Geometry: final body of the model. Coordinates: model frame, mm. A direction names the side the tool comes from. Round coordinates to 2 decimals unless told otherwise and drop trailing zeros. Loops run counter-clockwise (first coordinate to the right, second up) from the corner with the lowest first, then second, coordinate; pieces in that order, holes last. Notation, with made-up numbers: M 76.25,67.25 L 87.25,67.25 A32 ccw 87.25,97.25 Z; hole C 70.25,-20 d6. An arc over 180 degrees is marked long. Write each question's results on one line, items separated by ' | '.
Autodesk Inventor part; units mm, degrees
ref_plane "YZ Plane" through (0, 0, 0) normal (1, 0, 0) x (0, 1, 0)
ref_plane "XZ Plane" through (0, 0, 0) normal (0, 1, 0) x (-1, 0, 0)
ref_plane "XY Plane" through (0, 0, 0) normal (0, 0, 1) x (1, 0, 0)
sketch "Эскиз1" plane through (0, 0, 0) normal (0, 0, 1) x (1, 0, 0)
  line L0 (32.4057, 38.6485) -> (-32.4072, 38.6485)
  arc A0 (-32.4072, 38.6485) -> (-37.4072, 33.6485) centre (-32.4072, 33.6485) ccw
  line L1 (-37.4072, 33.6485) -> (-37.4072, 5)
  arc A1 (-37.4072, 5) -> (-32.4072, 0) centre (-32.4072, 5) ccw
  line L2 (-30, 0) -> (-29.5804, 0)
  arc A2 (-24.6503, -4.1667) -> (-29.5804, 0) centre (-29.5804, -5) ccw
  arc A3 (-24.6503, -4.1667) -> (24.6503, -4.1667) centre (0, 0) ccw
  arc A4 (29.5804, 0) -> (24.6503, -4.1667) centre (29.5804, -5) ccw
  circle A5 centre (0, 0) radius 13.45
  line L3 (-0.0007, 35) -> (-0.0007, -40.0249) construction
  line L4 (-31.1692, 11.8598) -> (-24.8192, 11.8598)
  line L5 (-24.8192, 11.8598) -> (-24.8192, 31.7098)
  line L6 (-24.8192, 31.7098) -> (-31.1692, 31.7098)
  line L7 (-31.1692, 31.7098) -> (-31.1692, 11.8598)
  line L8 (24.8177, 11.8598) -> (31.1677, 11.8598)
  line L9 (31.1677, 11.8598) -> (31.1677, 31.7098)
  line L10 (31.1677, 31.7098) -> (24.8177, 31.7098)
  line L11 (24.8177, 31.7098) -> (24.8177, 11.8598)
  arc A6 (37.4057, 33.6485) -> (32.4057, 38.6485) centre (32.4057, 33.6485) ccw
  line L12 (37.4057, 33.6485) -> (37.4057, 5)
  arc A7 (32.4057, 0) -> (37.4057, 5) centre (32.4057, 5) ccw
  line L13 (32.4057, 0) -> (29.5804, 0)
  line L14 (-32.4072, 0) -> (-30, 0)
  point P0 (29.9986, 30)
  point P1 (-30, 30)
  point P2 (25.9869, 30)
extrude "Выдавливание1" add sketch "Эскиз1" along normal blind 5
properties part number "Гор. шарнир"
1. Section A-A (x = 0). Output: boundary loops of the cut face in (y, z), then the cut area to 3 significant figures.
Answer key:
outline: M -25,0 L -13.45,0 L -13.45,5 L -25,5 Z; M 13.45,0 L 38.65,0 L 38.65,5 L 13.45,5 Z | area: 184 mm²
2. Section D-D (y = -11.5). Output: boundary loops of the cut face in (x, z), then the cut area to 3 significant figures.
Answer key:
outline: M -22.2,0 L -6.98,0 L -6.98,5 L -22.2,5 Z; M 6.98,0 L 22.2,0 L 22.2,5 L 6.98,5 Z | area: 152 mm²
3. Section C-C (y = 22). Output: boundary loops of the cut face in (x, z), then the cut area to 3 significant figures.
Answer key:
outline: M -37.41,0 L -31.17,0 L -31.17,5 L -37.41,5 Z; M -24.82,0 L 24.82,0 L 24.82,5 L -24.82,5 Z; M 31.17,0 L 37.41,0 L 37.41,5 L 31.17,5 Z | area: 311 mm²
4. Ray query, probe 1 along X at (y, z) = (29, 3.5); probe 2 along Y at (x, z) = (0, 3.5); probe 3 along Y at (x, z) = (5.5, 4.05). Return the intervals inside material, ascending.
Answer key:
probe 1: x = -37.41 to -31.17, -24.82 to 24.82, 31.17 to 37.41 | probe 2: y = -25 to -13.45, 13.45 to 38.65 | probe 3: y = -24.39 to -12.27, 12.27 to 38.65
5. Draft query along Y for faces 1 (the face through (35.902, 37.223, 2.465)), 2 (the face through (35.98, 1.504, 2.465)), 3 (the face through (31.168, 22, 2)). Return one class per face: pulls with the +Y half, pulls with the -Y half, needs draft (parallel to the pull), parting line crosses it, or undercut.
Answer key:
face 1: pulls with the +Y half | face 2: pulls with the -Y half | face 3: undercut
6. Section B-B (z = 4.1). Output: boundary loops of the cut face in (x, y), then the cut area to 3 significant figures.
Answer key:
outline: M -37.41,5 A5 ccw -32.41,0 L -29.58,0 A5 cw -24.65,-4.17 A25 ccw 24.65,-4.17 A5 cw 29.58,0 L 32.41,0 A5 ccw 37.41,5 L 37.41,33.65 A5 ccw 32.41,38.65 L -32.41,38.65 A5 ccw -37.41,33.65 Z; hole M -31.17,11.86 L -24.82,11.86 L -24.82,31.71 L -31.17,31.71 Z; hole C 0,0 d26.9; hole M 24.82,11.86 L 31.17,11.86 L 31.17,31.71 L 24.82,31.71 Z | area: 3,040 mm²
7. Access query for faces 4 (the face through (28, 31.71, 2)), 5 (the face through (-31, 0, 2)), 6 (the face through (31, 0, 2)). Directions: +Z, -Z, +X, -X, +Y, -Y. A direction counts if a zero-diameter tool reaches every point of the face in a straight line with its end or side. Return the directions, or none.
Answer key:
face 4: +Z, -Z | face 5: +Z, -Z, -X, -Y | face 6: +Z, -Z, +X, -Y
8. Pin query (flat end, axial travel): P1, Ø1.5, axis at x = -29, z = 2, coming from the -Y side; P2, Ø1.5, axis at x = 28, z = 2.5, coming from the -Y side; P3, Ø1, axis at y = -13, z = 3, coming from the +X side; P4, Ø24, axis at x = 0, y = 0, coming from the +Z side. Return the tip coordinate at first contact, or that it passes through.
Answer key:
P1: stops at y = -0.18 | P2: stops at y = -0.58 | P3: stops at x = 21.65 | P4: passes through
